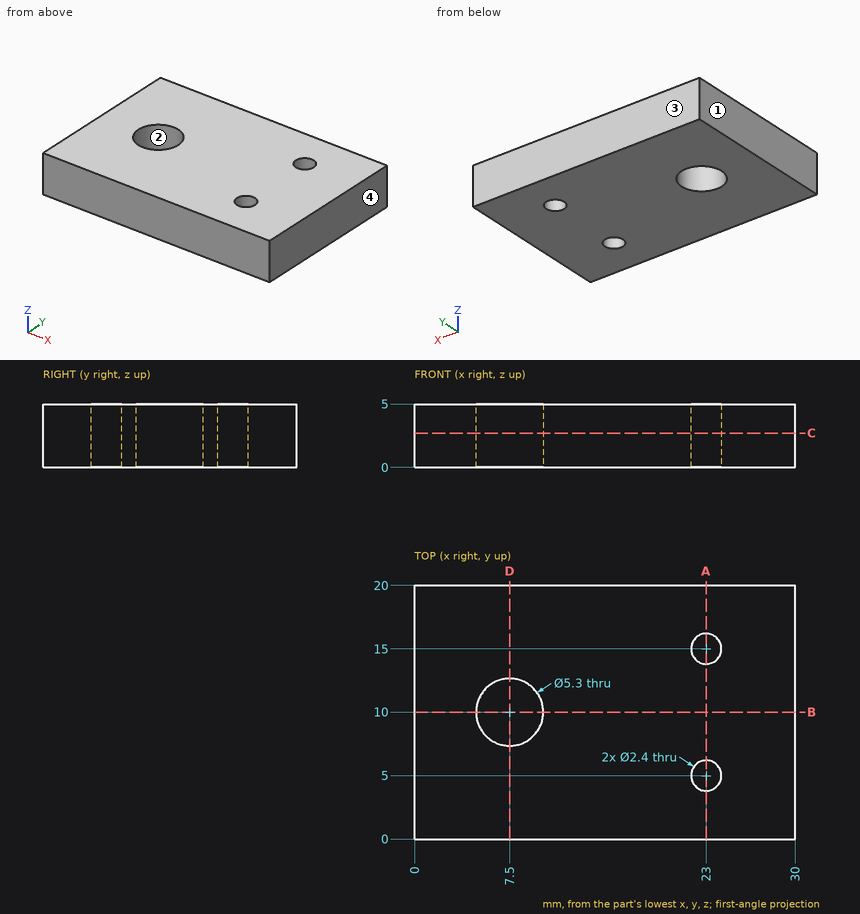
Print and shaded views of the part. All mm, measured from the part's lowest x, y and z. Coordinates: 2 decimals unless noted, no trailing zeros. Loops run counter-clockwise (first coordinate to the right, second up) from the corner with the lowest first, then second, coordinate; pieces in that order, holes last. Notation, with made-up numbers: (-22.75, 38.5) - (-14.75, 38.5) arc R13 cw to (-14.75, 47.5) - close; hole circle Ø3 at (33.25, 25). An arc over 180 degrees is marked (long way). Write item = value, one per line. Start each with the question number.
Item 1: Saw through at A-A, the plane x = 23. List the corners of the cut face in (y, z).
Item 2: Saw through at B-B, the plane y = 10. List the corners of the cut face in (x, z).
Item 3: Saw through at D-D, the plane x = 7.5. List the corners of the cut face in (y, z), then the cut area to 3 significant figures.
Item 4: Pull direction X, two halves, no side cores. Call the marked faces 1, 2, 3 and 4: +X half, -X half, draft (parallel to the pull), parting line (faces both ways), or undercut.
Item 5: Wall check: probe 1 along Y at (x, z) = (23, 3.25); probe 2 along Y at (x, z) = (7.5, 3.7); probe 3 along X at (y, z) = (14, 2.2). Give the ranges that are in metal, low to high. Write a range as [from, to].
Item 6: Saw through at C-C, the plane z = 2.7. List the corners of the cut face in (x, y).
Answers:
q1.outline = (0, 0) - (3.8, 0) - (3.8, 5) - (0, 5) - close; (6.2, 0) - (13.8, 0) - (13.8, 5) - (6.2, 5) - close; (16.2, 0) - (20, 0) - (20, 5) - (16.2, 5) - close
q2.outline = (0, 0) - (4.85, 0) - (4.85, 5) - (0, 5) - close; (10.15, 0) - (30, 0) - (30, 5) - (10.15, 5) - close
q3.outline = (0, 0) - (7.35, 0) - (7.35, 5) - (0, 5) - close; (12.65, 0) - (20, 0) - (20, 5) - (12.65, 5) - close
q3.area = 73.5 mm2
q4.face_1 = -X half
q4.face_2 = undercut
q4.face_3 = draft
q4.face_4 = +X half
q5.probe_1 = [0, 3.8], [6.2, 13.8], [16.2, 20]
q5.probe_2 = [0, 7.35], [12.65, 20]
q5.probe_3 = [0, 22.34], [23.66, 30]
q6.outline = (0, 0) - (30, 0) - (30, 20) - (0, 20) - close; hole circle Ø5.3 at (7.5, 10); hole circle Ø2.4 at (23, 5); hole circle Ø2.4 at (23, 15)
